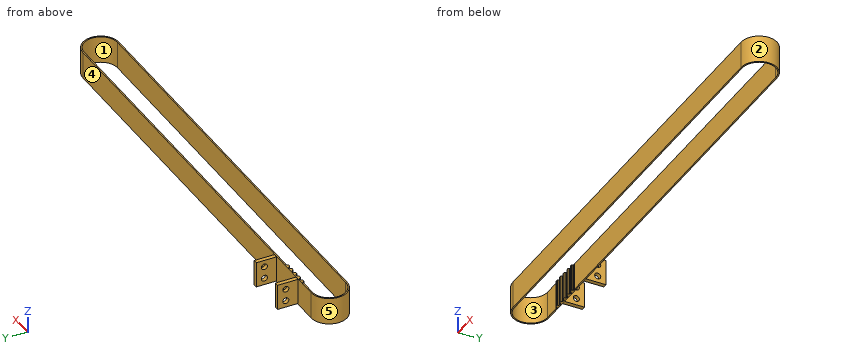
Autodesk Inventor part; units mm, degrees
ref_plane "作業平面3" through (140, 0, 0) normal (1, 0, 0) x (0, 1, 0)
ref_plane "作業平面6" through (140, 0, 0) normal (1, 0, 0) x (0, 1, 0)
ref_plane "XZ Plane" through (0, 0, 0) normal (0, 1, 0) x (-1, 0, 0)
sketch "Sketch_2" plane through (0, 0, 0) normal (0, 0, 1) x (1, 0, 0)
  arc A0 (-20, 13.3) -> (-20, -13.3) centre (-20, 0) ccw
  line L0 (-20, -13.3) -> (300, -13.3)
  arc A1 (300, -13.3) -> (300, 13.3) centre (300, 0) ccw
  line L1 (300, 13.3) -> (-20, 13.3)
extrude "Extrusion1" add sketch "Sketch_2" along normal mid plane 20
sketch "Sketch_8" plane through (0, 0, 0) normal (0, 0, 1) x (1, 0, 0)
  line L0 (-1.5, 28.3) -> (-1.5, 13.3)
  line L1 (-1.5, 13.3) -> (1.5, 13.3)
  line L2 (1.5, 13.3) -> (1.5, 28.3)
  line L3 (1.5, 28.3) -> (-1.5, 28.3)
extrude "Extrusion2" add sketch "Sketch_8" along normal mid plane 19
sketch "_____4" plane through (0, 0, 0) normal (1, 0, 0) x (0, 0, -1)
  circle A0 centre (-4.5, 22.3) radius 2.25
extrude "Extrusion3" cut sketch "_____4" along normal mid plane 6
sketch "_____5" plane through (0, 0, 0) normal (1, 0, 0) x (0, 0, -1)
  circle A0 centre (4.5, 22.3) radius 2.25
extrude "Extrusion4" cut sketch "_____5" along normal mid plane 6
sketch "_____2" plane through (0, 0, 0) normal (0, 0, 1) x (1, 0, 0)
  line L0 (28.5, 8.3) -> (31.5, 8.3)
  line L1 (31.5, 8.3) -> (31.5, 28.3)
  line L2 (31.5, 28.3) -> (28.5, 28.3)
  line L3 (28.5, 28.3) -> (28.5, 8.3)
extrude "Extrusion5" add sketch "_____2" along normal mid plane 19
sketch "Sketch6" plane through (28.5, 13.3, 9.5) normal (-1, 0, 0) x (0, 0, 1)
  point P0 (-14, 9)
hole "Hole1" at (28.5, 22.3, -4.5) direction (1, 0, 0) diameter 4.5 depth 3
sketch "Sketch7" plane through (28.5, 13.3, 9.5) normal (-1, 0, 0) x (0, 0, 1)
  point P0 (-5, 9)
hole "Hole2" at (28.5, 22.3, 4.5) direction (1, 0, 0) diameter 4.5 depth 3
sketch "Sketch_4" plane through (0, 0, 0) normal (0, 0, 1) x (1, 0, 0)
  arc A0 (-20, 12.3) -> (-20, -12.3) centre (-20, 0) ccw
  line L0 (-20, -12.3) -> (300, -12.3)
  arc A1 (300, -12.3) -> (300, 12.3) centre (300, 0) ccw
  line L1 (300, 12.3) -> (17.5, 12.3)
  line L2 (17.5, 12.3) -> (17.5, 11.1)
  line L3 (17.5, 11.1) -> (-7.5, 11.1)
  line L4 (-7.5, 11.1) -> (-7.5, 12.3)
  line L5 (-7.5, 12.3) -> (-20, 12.3)
extrude "Extrusion6" cut sketch "Sketch_4" along normal mid plane 20
sketch "Sketch_64" plane through (0, 0, 0) normal (0, 0, 1) x (1, 0, 0)
  line L0 (-9.3801, 11.1) -> (-9.3801, 10.1)
  line L1 (-9.3801, 10.1) -> (-5.6199, 10.1)
  line L2 (-5.6199, 10.1) -> (-5.6199, 11.1)
  arc A0 (-5.9958, 11.3632) -> (-5.6199, 11.1) centre (-5.6199, 11.5) ccw
  line L3 (-5.9958, 11.3632) -> (-6.241, 12.0368)
  arc A1 (-6.241, 12.0368) -> (-6.6168, 12.3) centre (-6.6168, 11.9) ccw
  line L4 (-6.6168, 12.3) -> (-7.125, 12.3)
  line L5 (-7.125, 12.3) -> (-7.125, 12.66)
  line L6 (-7.125, 12.66) -> (-7.875, 12.66)
  line L7 (-7.875, 12.66) -> (-7.875, 12.3)
  line L8 (-7.875, 12.3) -> (-8.3832, 12.3)
  arc A2 (-8.3832, 12.3) -> (-8.759, 12.0368) centre (-8.3832, 11.9) ccw
  line L9 (-8.759, 12.0368) -> (-9.0042, 11.3632)
  arc A3 (-9.3801, 11.1) -> (-9.0042, 11.3632) centre (-9.3801, 11.5) ccw
extrude "Extrusion7" cut sketch "Sketch_64" along normal mid plane 20
pattern_linear "Rectangular Pattern1" count 6 spacing 5 along (1, 0, 0) of "Extrusion7"
ref_plane "作業平面3" through (140, 0, 0) normal (1, 0, 0) x (0, 1, 0)
ref_plane "作業平面1" through (313.3, 0, 0) normal (1, 0, 0) x (0, 1, 0)
ref_plane "作業平面2" through (-33.3, 0, 0) normal (1, 0, 0) x (0, 1, 0)
ref_plane "作業平面6" through (140, 0, 0) normal (1, 0, 0) x (0, 1, 0)
ref_plane "作業平面4" through (313.3, 0, 0) normal (1, 0, 0) x (0, 1, 0)
ref_plane "作業平面5" through (-33.3, 0, 0) normal (1, 0, 0) x (0, 1, 0)
properties part number "ATBT-720T5200-B-P30_info-1-16-16"
Input: part model. Units: mm. Frame: model coordinates. Face numbers are marked on the shaded views. A direction names the side the tool comes from. Coordinates: 2 decimals unless noted, no trailing zeros. Write each loop counter-clockwise with the first axis right and the second up, starting at its lowest first coordinate (ties: lowest second). Pieces come first, ordered by that corner, then holes. Notation, with made-up numbers: (37, -6) -> (55, -6) arc R18 cw to (55, 13) -> close; hole circle Ø4 at (-5, 88). An arc over 180 degrees is marked (long way). Write each question's results on one line, items separated by ' | '.
Item 1: Pin query (flat end, axial travel): pin 1 Ø5 at (y, z) = (22.3, 4.5) entering from +X; pin 2 Ø3 at (y, z) = (-5, -3) entering from +X; pin 3 Ø4.5 at (y, z) = (17.5, 2.5) entering from -X. Return the tip coordinate at first contact, or that it passes through.
Conclusion:
pin 1: stops at x = 31.5 | pin 2: stops at x = 312.83 | pin 3: stops at x = -1.5
Item 2: Mould query, pull axis Y, two halves, no side actions, for the marked faces 3, 4 and 5. Classes: +Y half, -Y half, draft (parallel to the pull), parting line (faces both ways), or undercut.
Conclusion:
face 3: undercut | face 4: +Y half | face 5: parting line
Item 3: Section query A-A on x = 58.5. Return loops of the section in (y, z), plus the area to 3 significant figures.
Conclusion:
outline: (-13.3, -10) -> (-12.3, -10) -> (-12.3, 10) -> (-13.3, 10) -> close; (12.3, -10) -> (13.3, -10) -> (13.3, 10) -> (12.3, 10) -> close | area: 40.0 mm^2
Item 4: Set-up query: the marked faces 1 and 2. Return all of +Z, -Z, +X, -X, +Y, -Y with unobstructed straight access to the full face (end or side cutting, diameter ignored); none if empty.
Conclusion:
face 1: +Z, -Z | face 2: +Z, -Z, +X
Item 5: Section query B-B on y = -5. Return loops of the section in (x, z).
Conclusion:
outline: (-32.32, -10) -> (-31.24, -10) -> (-31.24, 10) -> (-32.32, 10) -> close; (311.24, -10) -> (312.32, -10) -> (312.32, 10) -> (311.24, 10) -> close
Item 6: Material intervals for probe 1 along Y at (x, z) = (29.7, 4.5); probe 2 along Z at (x, y) = (0, 22); probe 3 along Y at (x, z) = (-0.6, 4.5), sorted ascending.
Conclusion:
probe 1: y = -13.3 to -12.3, 12.3 to 20.05, 24.55 to 28.3 | probe 2: z = -9.5 to -6.73, -2.27 to 2.27, 6.73 to 9.5 | probe 3: y = -13.3 to -12.3, 11.1 to 20.05, 24.55 to 28.3
